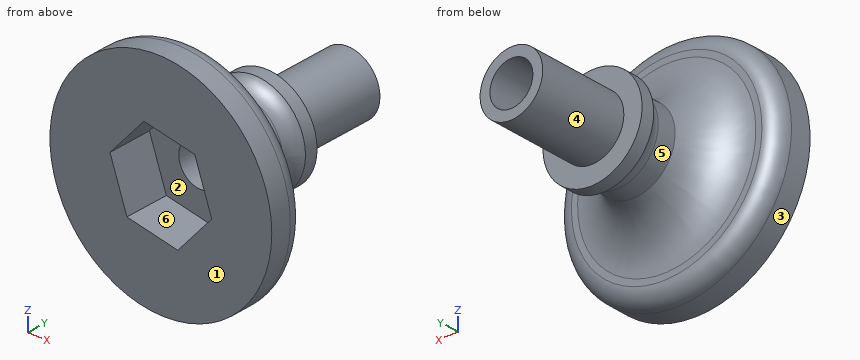
Autodesk Inventor part; units mm, degrees
ref_plane "YZ Plane" through (0, 0, 0) normal (1, 0, 0) x (0, 1, 0)
ref_plane "XZ Plane" through (0, 0, 0) normal (0, 1, 0) x (-1, 0, 0)
ref_plane "XY Plane" through (0, 0, 0) normal (0, 0, 1) x (1, 0, 0)
sketch "Sketch1" plane through (0, 0, 0) normal (1, 0, 0) x (0, 1, 0)
  line L0 (0, 0) -> (0, -10.795)
  line L1 (0, -10.795) -> (2.54, -10.795)
  line L2 (0, 0) -> (12.7, 0)
  line L3 (2.54, -10.795) -> (2.54, -9.9414)
  line L4 (2.54, -9.9414) -> (2.54, -8.6714)
  line L5 (14.986, -3.937) -> (1.8235, -3.937) construction
  arc A0 (6.0461, -3.937) -> (2.54, -8.6714) centre (7.4896, -8.6714) ccw
  line L6 (9.398, -3.048) -> (9.398, -4.826)
  line L7 (6.0461, -3.937) -> (7.8921, -3.937)
  arc A1 (9.398, -4.826) -> (7.8921, -3.937) centre (7.8921, -5.6569) ccw
  line L8 (19.558, 0) -> (0, 0)
  line L9 (9.398, -3.048) -> (19.558, -3.048)
  line L10 (19.558, -3.048) -> (19.558, 0)
  dimension "d0" = 10.795
  dimension "d1" = 2.54
  dimension "d2" = 12.7
  dimension "d5" = 3.937
  dimension "d6" = 1.27
  dimension "d7" = 4.9496
  dimension "d18" = 4.826
  dimension "d19" = 1.7199
  dimension "d24" = 9.398
  dimension "d25" = 10.16
  dimension "d26" = 3.048
  dimension "d27" = 4.572
  dimension "d28" = 5.6234
  dimension "d29" = 17.7345
revolve "Revolution1" add sketch "Sketch1" angle 360 about axis through (0, 0, 0) along (0, 1, 0)
sketch "Sketch2" plane through (0, 0, 0) normal (0, -1, 0) x (1, 0, 0)
  circle A0 centre (0, 0) radius 3.048
  line L0 (4.95, -0.9536) -> (1.6491, -4.7636)
  line L1 (1.6491, -4.7636) -> (-3.3008, -3.81)
  line L2 (-3.3008, -3.81) -> (-4.95, 0.9536)
  line L3 (-4.95, 0.9536) -> (-1.6491, 4.7636)
  line L4 (-1.6491, 4.7636) -> (3.3008, 3.81)
  line L5 (3.3008, 3.81) -> (4.95, -0.9536)
  dimension "d11" = 8.7312
  dimension "d12" = 7.62
extrude "Extrusion1" cut sketch "Sketch2" against normal blind 3.302 contours A0 | L0 L1 L2 L3 L4 L5
sketch "Sketch3" plane through (0, 3.302, 0) normal (0, -1, 0) x (1, 0, 0)
  circle A0 centre (0, 0) radius 2.0892
  dimension "d15" = 4.1783
extrude "Extrusion2" cut sketch "Sketch3" against normal up to surface (16.256 mm away)
sketch "Sketch5" plane through (0, 9.398, 0) normal (0, 1, 0) x (1, 0, 0)
  circle A0 centre (0, 0) radius 4.826
  circle A1 centre (0, 0) radius 3.048
extrude "Extrusion5" add sketch "Sketch5" along normal blind 1.27
sketch "Sketch6" plane through (0, 0, 0) normal (0, -1, 0) x (1, 0, 0)
  circle A0 centre (0, 0) radius 10.795
  line L0 (3.3008, 3.81) -> (4.95, -0.9536)
  line L1 (4.95, -0.9536) -> (1.6491, -4.7636)
  line L2 (1.6491, -4.7636) -> (-3.3008, -3.81)
  line L3 (-3.3008, -3.81) -> (-4.95, 0.9536)
  line L4 (-4.95, 0.9536) -> (-1.6491, 4.7636)
  line L5 (-1.6491, 4.7636) -> (3.3008, 3.81)
extrude "Extrusion6" add sketch "Sketch6" along normal blind 1.016
fillet "Fillet1" radius 1.524 1 edges at (0, 2.54, 10.795)
properties part number "_3DPrint"
Model file for the job. Use its own axes, mm. Face numbers are marked on the shaded views. A direction names the side the tool comes from. Coordinates: 2 decimals unless noted, no trailing zeros. Order: outer loops, then holes, each group sorted by start corner. A loop starts at its lowest first (then second) coordinate and runs counter-clockwise, first axis right, second up. Notation, with made-up numbers: (-28.75, -18.5) - (18.25, -18.5) arc R15 ccw to (18.25, -2.5) - close; hole circle Ø1 at (50.25, -3). An arc over 180 degrees is marked (long way). Return JSON: item names as keys, results as strings. Group by question number.
1) Flat gauge pins, fed straight in: P1, Ø10, axis at x = 3.5, y = 14, coming from the -Z side; P2, Ø4, axis at x = -0.5, y = 10, coming from the +Z side; P3, Ø3, axis at x = -1.5, z = 1, coming from the -Y side. Where does each tip first touch, or does it go through?
2) Saw through at A-A, the plane x = 0. Write the cut outline in (y, z) (3 decimals), plus the area to 3 significant figures.
3) Probe line 1 (Z direction, x = 0, y = 9.5); line 2 (Z direction, x = 0, y = 8); line 3 (Y direction, x = -1.5, z = -5). List the from-to ranges inside material, lowest first. Write a range as from..to.
4) Tool access for the marked faces 4, 5 and 6: list every direction of +Z, -Z, +X, -X, +Y, -Y with a clear straight run to the whole face (end or side of a thin tool).
5) Saw through at B-B, the plane z = 0. Write the cut outline in (x, y) (3 decimals).
6) Mould opens along Z. For the marked faces 1, 2 and 3 say: released by +Z, released by -Z, zero draft, split by the parting line, or undercut.
Values found:
{
 "1": {"P1": "stops at z = -4.83", "P2": "stops at z = 4.83", "P3": "stops at y = 3.3"},
 "2": {"outline": "(-1.016, -10.795) - (1.016, -10.795) arc R1.524 ccw to (2.54, -9.271) - (2.54, -8.671) arc R4.95 cw to (6.046, -3.937) - (7.892, -3.937) arc R1.72 cw to (9.398, -4.826) - (10.668, -4.826) - (10.668, -3.048) - (19.558, -3.048) - (19.558, -2.089) - (3.302, -2.089) - (3.302, -4.446) - (-1.016, -4.446) - close; (-1.016, 4.446) - (3.302, 4.446) - (3.302, 2.089) - (19.558, 2.089) - (19.558, 3.048) - (10.668, 3.048) - (10.668, 4.826) - (9.398, 4.826) arc R1.72 cw to (7.892, 3.937) - (6.046, 3.937) arc R4.95 cw to (2.54, 8.671) - (2.54, 9.271) arc R1.524 ccw to (1.016, 10.795) - (-1.016, 10.795) - close", "area": "99.5 mm²"},
 "3": {"line 1": "z = -4.83..-2.09, 2.09..4.83", "line 2": "z = -3.94..-2.09, 2.09..3.94", "line 3": "y = -1.02..3.94"},
 "4": {"face 4": "+Y", "face 5": "none", "face 6": "-Y"},
 "5": {"outline": "(-10.795, -1.016) - (-4.62, -1.016) - (-4.62, 3.302) - (-2.089, 3.302) - (-2.089, 19.558) - (-3.048, 19.558) - (-3.048, 10.668) - (-4.826, 10.668) - (-4.826, 9.398) arc R1.72 cw to (-3.937, 7.892) - (-3.937, 6.046) arc R4.95 cw to (-8.671, 2.54) - (-9.271, 2.54) arc R1.524 ccw to (-10.795, 1.016) - close; (2.089, 3.302) - (4.62, 3.302) - (4.62, -1.016) - (10.795, -1.016) - (10.795, 1.016) arc R1.524 ccw to (9.271, 2.54) - (8.671, 2.54) arc R4.95 cw to (3.937, 6.046) - (3.937, 7.892) arc R1.72 cw to (4.826, 9.398) - (4.826, 10.668) - (3.048, 10.668) - (3.048, 19.558) - (2.089, 19.558) - close"},
 "6": {"face 1": "zero draft", "face 2": "undercut", "face 3": "split by the parting line"}
}
